Work out the finished part from the listing and answer in its coordinate system (mm). Give positions to 0.01 mm unless a question says otherwise; leave off trailing zeros. Order: outer loops, then holes, each group sorted by start corner. A loop starts at its lowest first (then second) coordinate and runs counter-clockwise, first axis right, second up. Notation, with made-up numbers: M 21,63.5 L 33,63.5 A19 cw 33,95.5 Z; hole C 48,-36.75 d5. An arc over 180 degrees is marked long. One line per item, written item: value.
from build123d import *

# Parameters (mm, degrees)
F0_R     = 6.35
F1_DEPTH = 0.64516


with BuildPart() as f1:
    # F0 (on Front) → F1 (new body)
    with BuildSketch(Plane.XZ):
        with BuildLine():
            ThreePointArc((0, 1.27), (0.371974, 0.371974), (1.27, 0))
            Line((1.27, 0), (119.38, 0))
            ThreePointArc((119.38, 0), (120.278026, 0.371974), (120.65, 1.27))
            Line((120.65, 1.27), (120.65, 8.255))
            ThreePointArc((120.65, 8.255), (121.021974, 9.153026), (121.92, 9.525))
            Line((121.92, 9.525), (150.495, 9.525))
            ThreePointArc((150.495, 9.525), (156.332166, 11.942834), (158.75, 17.78))
            Line((158.75, 17.78), (158.75, 36.195))
            ThreePointArc((158.75, 36.195), (156.332166, 42.032166), (150.495, 44.45))
            Line((150.495, 44.45), (142.54871, 44.45))
            ThreePointArc((142.54871, 44.45), (135.497057, 44.123014), (128.505923, 43.144861))
            Line((128.505923, 43.144861), (1.035954, 19.244241))
            ThreePointArc((1.035954, 19.244241), (0.292723, 18.807061), (0, 17.995994))
            Line((0, 17.995994), (0, 1.27))
        make_face()
        with Locations((139.7, 28.575)):
            Circle(F0_R, mode=Mode.SUBTRACT)
    extrude(amount=F1_DEPTH)


solid = f1.part
(1) Find the intervals of material crossed by probe 1 along Z at (x, y) = (139.7, -0.35) (3 decimals); probe 2 along X at (y, z) = (-0.05, 3); probe 3 along Z at (x, y) = (54, -0.25) (3 decimals), in increasing order. Write a range as from..to.
Findings:
probe 1: z = 9.525..22.225, 34.925..44.397
probe 2: x = 0..120.65
probe 3: z = 0..29.175
(2) Determine the mould class of faces 1 (the cylindrical face through (134.66, -0.32, 24.71)), 2 (the flat face through (78, -0.645, 18)), 3 (the flat face through (65.66, -0.32, 31.36)) for opening direction Z: pulls with the +Z half, pulls with the -Z half, needs draft (parallel to the pull), parting line crosses it, or undercut.
Findings:
face 1: undercut
face 2: needs draft
face 3: pulls with the +Z half
(3) Section A-A, the plane y = -0.2 is taken. Give the vertices of the cut face in (x, z) (3 decimals), then the cut area to 3 significant figures.
Findings:
outline: M 0,1.27 A1.27 ccw 1.27,0 L 119.38,0 A1.27 ccw 120.65,1.27 L 120.65,8.255 A1.27 cw 121.92,9.525 L 150.495,9.525 A8.255 ccw 158.75,17.78 L 158.75,36.195 A8.255 ccw 150.495,44.45 L 142.549,44.45 A76.2 ccw 128.506,43.145 L 1.036,19.244 A1.27 ccw 0,17.996 Z; hole C 139.7,28.575 d12.7
area: 4,820 mm^2
(4) Section B-B, the plane x = 139.7 is taken. Give the vertices of the cut face in (y, z) (3 decimals), then the cut area to 3 significant figures.
Findings:
outline: M -0.645,9.525 L 0,9.525 L 0,22.225 L -0.645,22.225 Z; M -0.645,34.925 L 0,34.925 L 0,44.397 L -0.645,44.397 Z
area: 14.3 mm^2
(5) Section C-C, the plane z = 11 is taken. Give the vertices of the cut face in (x, y), then the cut area to 3 significant figures.
Findings:
outline: M 0,-0.65 L 155.2,-0.65 L 155.2,0 L 0,0 Z
area: 100 mm^2
(6) Given P1, Ø11.5, axis at x = 139.7, z = 28.575, coming from the +Y side; P2, Ø1.5, axis at x = 34, z = 19.5, coming from the +Y side, each flat-ended and moving along its own axis, determine where each tip first touches the part or whether it passes through.
Findings:
P1: passes through
P2: stops at y = 0
(7) Section D-D, the plane x = 97.5 is taken. Give the vertices of the cut face in (y, z), then the cut area to 3 significant figures.
Findings:
outline: M -0.65,0 L 0,0 L 0,37.33 L -0.65,37.33 Z
area: 24.1 mm^2
